Check sheet for the modelled part. Datum: model origin and axes. Units: mm. Face numbers are marked on the shaded views. Coordinates: 2 decimals unless noted, no trailing zeros. Write each loop counter-clockwise with the first axis right and the second up, starting at its lowest first coordinate (ties: lowest second). Pieces come first, ordered by that corner, then holes. Notation, with made-up numbers: (62, -7.5) -> (75, -7.5) arc R21 cw to (75, 8.5) -> close; hole circle Ø8 at (-17.75, -33). An arc over 180 degrees is marked (long way). Put each result on its own line as item: value.
```python
from build123d import *

# Parameters (mm, degrees)
CYLINDER_R        = 6
CYLINDER_DEPTH    = 9
SKETCH_R          = 1.25
POCKET_DEPTH      = 3
CYLINDER002_R     = 0.3
CYLINDER002_DEPTH = 5
CYLINDER001_R     = 0.3
CYLINDER001_DEPTH = 7


with BuildPart() as hole_pocket:
    # Cylinder → Cylinder (new body)
    with BuildSketch(Plane.XY):
        Circle(CYLINDER_R)
    extrude(amount=CYLINDER_DEPTH)

    # Sketch → Pocket (cut)
    with BuildSketch(Plane.XY.offset(9)):
        Circle(SKETCH_R)
    extrude(amount=-POCKET_DEPTH, mode=Mode.SUBTRACT)


with BuildPart() as cathode_cylinder:
    # Cylinder002 → Cylinder002 (new body)
    with BuildSketch(Plane(origin=(3.75, 0, -5), x_dir=(1, 0, 0), z_dir=(0, 0, 1))):
        Circle(CYLINDER002_R)
    extrude(amount=CYLINDER002_DEPTH)


with BuildPart() as buzzer:
    # Cylinder001 → Cylinder001 (new body)
    with BuildSketch(Plane(origin=(-3.75, 0, -7), x_dir=(1, 0, 0), z_dir=(0, 0, 1))):
        Circle(CYLINDER001_R)
    extrude(amount=CYLINDER001_DEPTH)

    # Fusion: union hole-pocket, cathode-cylinder
    add(hole_pocket.part)
    add(cathode_cylinder.part)


solid = buzzer.part
```
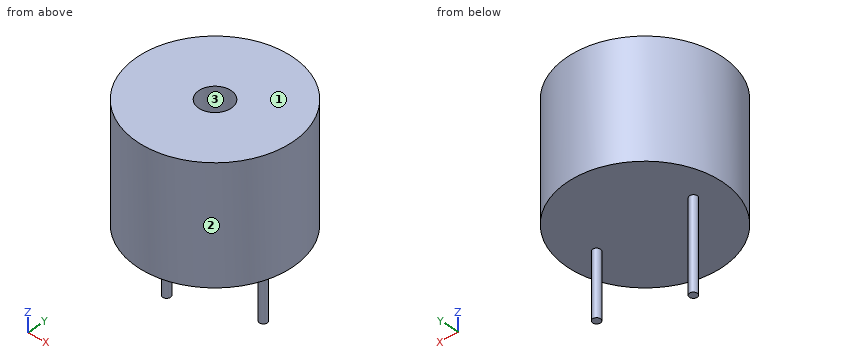
Q1. Mould release check, pull along X, two halves, no side actions. Record for the marked faces 1, 2 and 3: released by +X, released by -X, zero draft, split by the parting line, or undercut.
Recorded:
face 1: zero draft
face 2: split by the parting line
face 3: undercut
Q2. Cross-section at C-C (z = 6.5). Record the cut outline in (x, y).
Recorded:
outline: circle Ø12 at (0, 0); hole circle Ø2.5 at (0, 0)
Q3. Cross-section at A-A (x = 0). Record the cut outline in (y, z).
Recorded:
outline: (-6, 0) -> (6, 0) -> (6, 9) -> (1.25, 9) -> (1.25, 6) -> (-1.25, 6) -> (-1.25, 9) -> (-6, 9) -> close
Q4. Material ranges on line 1 along Y through (x, z) = (0, 7.5); line 2 along Z through (x, y) = (4, 0.25); line 3 along Y through (x, z) = (0.25, 5.5), recorded low to high.
Recorded:
line 1: y = -6 to -1.25, 1.25 to 6
line 2: z = 0 to 9
line 3: y = -5.99 to 5.99
Q5. Depth check by flat-ended pin: P1, Ø1, axis at x = -3.5, z = 6, coming from the +Y side; P2, Ø0.8, axis at x = 0.5, y = -0.5, coming from the +Z side; P3, Ø2, axis at y = 1, z = -5, coming from the +X side. Enter the tip coordinate at first touch or a pass-through.
Recorded:
P1: stops at y = 5.2
P2: stops at z = 6
P3: stops at x = 4.05
Q6. Cross-section at D-D (x = -3.75). Record the cut outline in (y, z), plus the area to 3 significant figures.
Recorded:
outline: (-4.68, 0) -> (-0.3, 0) -> (-0.3, -7) -> (0.3, -7) -> (0.3, 0) -> (4.68, 0) -> (4.68, 9) -> (-4.68, 9) -> close
area: 88.5 mm2
Q7. Cross-section at B-B (y = 0). Record the cut outline in (x, z).
Recorded:
outline: (-6, 0) -> (-4.05, 0) -> (-4.05, -7) -> (-3.45, -7) -> (-3.45, 0) -> (3.45, 0) -> (3.45, -5) -> (4.05, -5) -> (4.05, 0) -> (6, 0) -> (6, 9) -> (1.25, 9) -> (1.25, 6) -> (-1.25, 6) -> (-1.25, 9) -> (-6, 9) -> close
